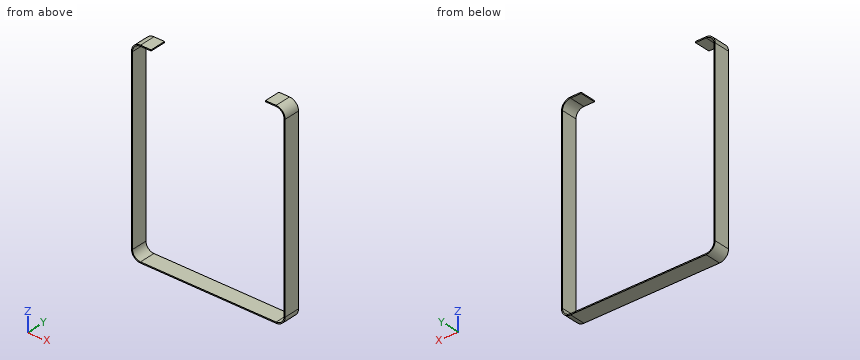
Autodesk Inventor part; units mm, degrees
ref_plane "YZ Plane" through (0, 0, 0) normal (1, 0, 0) x (0, 1, 0)
ref_plane "XZ Plane" through (0, 0, 0) normal (0, 1, 0) x (-1, 0, 0)
ref_plane "XY Plane" through (0, 0, 0) normal (0, 0, 1) x (1, 0, 0)
sketch "Sketch1" plane through (0, 0, 0) normal (0, 1, 0) x (-1, 0, 0)
  line L0 (0, 0) -> (-361.95, 0)
  line L1 (-361.95, 0) -> (-361.95, -463.55)
  line L2 (-361.95, -463.55) -> (0, -463.55)
  line L3 (0, -463.55) -> (0, 0)
  dimension "d0" = 361.95
  dimension "d1" = 463.55
extrude "Extrusion1" add sketch "Sketch1" along normal blind 2.794
fillet "Fillet1" radius 19.05 4 edges at (361.95, 1.397, 0) (361.95, 1.397, -463.55) (0, 1.397, -463.55) (0, 1.397, 0)
sketch "Sketch2" plane through (0, 0, 0) normal (0, -1, 0) x (1, 0, 0)
  line L0 (19.05, 0) -> (342.9, 0)
  line L1 (342.9, 0) -> (342.9, -2.8525)
  line L2 (342.9, -2.8525) -> (19.05, -2.8525)
  line L3 (19.05, -2.8525) -> (19.05, 0)
  line L4 (342.9, -2.8525) -> (317.5, -2.8525)
  line L5 (317.5, -2.8525) -> (317.5, 0)
  line L6 (317.5, 0) -> (342.9, 0)
  line L7 (342.9, 0) -> (342.9, -2.8525)
  line L8 (19.05, -2.8525) -> (44.45, -2.8525)
  line L9 (44.45, -2.8525) -> (44.45, 0)
  line L10 (44.45, 0) -> (19.05, 0)
  line L11 (19.05, 0) -> (19.05, -2.8525)
  line L12 (44.45, -2.8525) -> (317.5, -2.8525)
  line L13 (317.5, -2.8525) -> (317.5, 0)
  line L14 (317.5, 0) -> (44.45, 0)
  line L15 (44.45, 0) -> (44.45, -2.8525)
  point P0 (0, 0)
  dimension "d5" = 25.4
  dimension "d6" = 25.4
extrude "Extrusion2" add sketch "Sketch2" along normal blind 25.4 contours L0 L5 L2 L9
sketch "Sketch3" plane through (19.05, 2.794, 0) normal (0, 0, 1) x (1, 0, 0)
  line L0 (323.85, -2.794) -> (0, -2.794)
  line L1 (25.405, -2.794) -> (25.4, -15.494)
  line L2 (25.4, -2.794) -> (25.4, -28.194)
  line L3 (25.4, -15.494) -> (85.4, -15.5178)
  line L4 (298.45, -2.794) -> (298.45, -28.194)
  line L5 (298.45, -15.494) -> (238.45, -15.494)
  circle A0 centre (85.4, -15.5178) radius 3.429
  circle A1 centre (238.45, -15.494) radius 3.429
  point P0 (-19.05, -2.794)
  dimension "d9" = 12.7
  dimension "d10" = 60
  dimension "d11" = 60
  dimension "d12" = 6.858
  dimension "d13" = 6.858
extrude "Extrusion3" cut sketch "Sketch3" against normal blind 25.4 contours A0 | A1
sketch "Sketch4" plane through (0, 2.794, 0) normal (0, 1, 0) x (1, 0, 0)
  arc A0 (0, 19.05) -> (19.05, 0) centre (19.05, 19.05) ccw
  line L0 (19.05, 0) -> (342.9, 0)
  arc A1 (342.9, 0) -> (361.95, 19.05) centre (342.9, 19.05) ccw
  line L1 (361.95, 19.05) -> (361.95, 444.5)
  arc A2 (361.95, 444.5) -> (342.9, 463.55) centre (342.9, 444.5) ccw
  line L2 (342.9, 463.55) -> (19.05, 463.55)
  arc A3 (19.05, 463.55) -> (0, 444.5) centre (19.05, 444.5) ccw
  line L3 (0, 444.5) -> (0, 19.05)
  arc A4 (-2.54, 19.05) -> (19.05, -2.54) centre (19.05, 19.05) ccw
  line L4 (19.05, -2.54) -> (342.9, -2.54)
  arc A5 (342.9, -2.54) -> (364.49, 19.05) centre (342.9, 19.05) ccw
  line L5 (364.49, 19.05) -> (364.49, 444.5)
  arc A6 (364.49, 444.5) -> (342.9, 466.09) centre (342.9, 444.5) ccw
  line L6 (342.9, 466.09) -> (19.05, 466.09)
  arc A7 (19.05, 466.09) -> (-2.54, 444.5) centre (19.05, 444.5) ccw
  line L7 (-2.54, 444.5) -> (-2.54, 19.05)
  line L8 (44.45, 0) -> (44.45, -2.54)
  line L9 (317.5, 0) -> (317.5, -2.54)
  point P0 (0, 0)
  dimension "d16" = 2.54
extrude "Extrusion4" add sketch "Sketch4" along normal blind 38.1 contours A0 L0 L8 L4 A4 L7 A7 L6 A6 L5 A5 L9 A1 L1 A2 L2 A3 L3
sketch "Sketch5" plane through (0, 2.794, 0) normal (0, 1, 0) x (1, 0, 0)
  arc A0 (0, 19.05) -> (19.05, 0) centre (19.05, 19.05) ccw
  line L0 (19.05, 0) -> (44.45, 0)
  line L1 (44.45, 0) -> (317.5, 0)
  line L2 (317.5, 0) -> (342.9, 0)
  arc A1 (342.9, 0) -> (361.95, 19.05) centre (342.9, 19.05) ccw
  line L3 (361.95, 19.05) -> (361.95, 444.5)
  arc A2 (361.95, 444.5) -> (342.9, 463.55) centre (342.9, 444.5) ccw
  line L4 (342.9, 463.55) -> (19.05, 463.55)
  arc A3 (19.05, 463.55) -> (0, 444.5) centre (19.05, 444.5) ccw
  line L5 (0, 444.5) -> (0, 19.05)
  point P0 (0, 0)
extrude "Extrusion5" cut sketch "Sketch5" against normal blind 38.1
properties part number "Cart_TOP_SHELF-LIP" material "Cart Material"
Input: part model. Units: mm. Frame: model coordinates. Round coordinates to 2 decimals unless told otherwise and drop trailing zeros. Order: outer loops, then holes, each group sorted by start corner. A loop starts at its lowest first (then second) coordinate and runs counter-clockwise, first axis right, second up. Notation, with made-up numbers: (-12.75, 38) - (2.25, 38) arc R7 cw to (2.25, 47) - close; hole circle Ø9 at (45.25, -4). An arc over 180 degrees is marked (long way). One line per question, with ' | ' between items. Start each with the question number.
1) Cut plane A-A, the plane z = -170. Return the cut outline in (x, y).
2) Contact query for flat-ended pins moving along their axis: P1, Ø1.3, axis at y = 18.5, z = 1.5, coming from the -X side; P2, Ø1, axis at x = 84.5, y = 24.5, coming from the +Z side; P3, Ø3, axis at y = 31, z = 0.5, coming from the +X side. Output: stop coordinate, or through.
3) Cut plane B-B, the plane y = 19. Return the cut outline in (x, z), then the cut area to 3 significant figures.
4) Cut plane C-C, the plane x = 242.5. Return the cut outline in (y, z).
5) Ray query, probe 1 along X at (y, z) = (20.5, -96.5); probe 2 along Z at (x, y) = (320.5, 8); probe 3 along Z at (x, y) = (228.5, 4.5). Return the intervals inside material, ascending.
Worked out:
1) outline: (-2.54, 2.79) - (0, 2.79) - (0, 40.89) - (-2.54, 40.89) - close; (361.95, 2.79) - (364.49, 2.79) - (364.49, 40.89) - (361.95, 40.89) - close
2) P1: stops at x = 10.68 | P2: stops at z = -463.55 | P3: stops at x = 354.75
3) outline: (-2.54, -444.5) arc R21.59 ccw to (19.05, -466.09) - (342.9, -466.09) arc R21.59 ccw to (364.49, -444.5) - (364.49, -19.05) arc R21.59 ccw to (342.9, 2.54) - (317.5, 2.54) - (317.5, 0) - (342.9, 0) arc R19.05 cw to (361.95, -19.05) - (361.95, -444.5) arc R19.05 cw to (342.9, -463.55) - (19.05, -463.55) arc R19.05 cw to (0, -444.5) - (0, -19.05) arc R19.05 cw to (19.05, 0) - (44.45, 0) - (44.45, 2.54) - (19.05, 2.54) arc R21.59 ccw to (-2.54, -19.05) - close | area: 3,440 mm^2
4) outline: (2.79, -466.09) - (40.89, -466.09) - (40.89, -463.55) - (2.79, -463.55) - close
5) probe 1: x = -2.54 to 0, 361.95 to 364.49 | probe 2: z = -466.09 to -463.55, 0 to 2.54 | probe 3: z = -466.09 to -463.55
